```python
from build123d import *

# Parameters (mm, degrees)
HOLE_WIZARD_4_0_2_D     = 4
HOLE_WIZARD_4_0_2_DEPTH = 5
HOLE_WIZARD_4_0_2_TIP   = 1.201721238


with BuildPart() as part:
    # Эскиз1 → Повернуть1 (revolve)
    with BuildSketch(Plane.XY):
        Polygon((1.5, 18.5), (8.5, 18.5), (10, 20), (10, 24.5), (8.5, 26), (1.5, 26), (0, 24.5), (0, 20), align=None)
    revolve(axis=Axis((0, 0, 0), (1, 0, 0)))

    # Отверстия под штифты Ø4.0 мм2
    with Locations(Plane.ZY):
        with Locations((-22, 0), (0, 22), (22, 0), (0, -22)):
            Hole(HOLE_WIZARD_4_0_2_D / 2, depth=HOLE_WIZARD_4_0_2_DEPTH)
            with Locations((0, 0, -(HOLE_WIZARD_4_0_2_DEPTH + HOLE_WIZARD_4_0_2_TIP / 2))):  # 118° drill point
                Cone(0, HOLE_WIZARD_4_0_2_D / 2, HOLE_WIZARD_4_0_2_TIP, mode=Mode.SUBTRACT)


solid = part.part
```
CAD build for the part. Positions are in the model's coordinates, mm. A direction names the side the tool comes from. Give positions to 0.01 mm unless a question says otherwise; leave off trailing zeros. Write each loop counter-clockwise with the first axis right and the second up, starting at its lowest first coordinate (ties: lowest second). Pieces come first, ordered by that corner, then holes. Notation, with made-up numbers: (71.25, 17) -> (77.25, 17) arc R9 cw to (77.25, 26) -> close; hole circle Ø6 at (30.5, 7.5). An arc over 180 degrees is marked (long way). Write each question's results on one line, items separated by ' | '.
1. Wall check: probe 1 along Z at (x, y) = (3.5, 0); probe 2 along Y at (x, z) = (2, 7.5); probe 3 along Z at (x, y) = (1.7, 22). Give the ranges that are in metal, low to high. Write a range as [from, to].
Geometry check:
probe 1: [-26, -24], [-20, -18.5], [18.5, 20], [24, 26] | probe 2: [-24.89, -16.91], [16.91, 24.89] | probe 3: [-13.86, -2], [2, 13.86]
2. Two-plate mould, pull along Y, no slides. Class faces 1 (the flat face through (10, 9.2, -18)), 2 (the cylindrical face through (4.951, -20.633, -15.821)), 3 (the cylindrical face through (5.05, -4.01, -18.06)): pulls with the +Y half, pulls with the -Y half, needs draft (parallel to the pull), parting line crosses it, or undercut.
Geometry check:
face 1: needs draft | face 2: parting line crosses it | face 3: undercut
3. Drop flat-ended pins along their axis: P1, Ø5, axis at x = 6.5, y = 14.5, coming from the -Z side; P2, Ø6, axis at x = 6, z = 14, coming from the -Y side; P3, Ø1, axis at x = 2, y = 8, coming from the +Z side. Give the stop position or say it passes through.
Geometry check:
P1: z = -23.07 | P2: y = -23.56 | P3: z = 24.89
4. Cut at B-B, the plane x = 7.75. Write the cut outline in (y, z), then the cut area to 3 significant figures.
Geometry check:
outline: circle Ø52 at (0, 0); hole circle Ø37 at (0, 0) | area: 1,050 mm²
5. Which spindle directions (+Z, -Z, +X, -X, +Y, -Y) get a long thin tool onto all of the face, cutting with end or side? Do faces 4 (the cylindrical face through (2.5, -1.2, 23.6)), 5 (the flat face through (0, 4, -20)). Say none if no direction does.
Geometry check:
face 4: -X | face 5: +Z, -Z, -X, +Y, -Y
6. Cut at A-A, the plane y = 0. Write the cut outline in (x, z).
Geometry check:
outline: (0, -24.5) -> (1.5, -26) -> (8.5, -26) -> (10, -24.5) -> (10, -20) -> (8.5, -18.5) -> (1.5, -18.5) -> (0, -20) -> (5, -20) -> (6.2, -22) -> (5, -24) -> (0, -24) -> close; (0, 20) -> (1.5, 18.5) -> (8.5, 18.5) -> (10, 20) -> (10, 24.5) -> (8.5, 26) -> (1.5, 26) -> (0, 24.5) -> (0, 24) -> (5, 24) -> (6.2, 22) -> (5, 20) -> close
